```python
from build123d import *

# Parameters (mm, degrees)
F0_R      = 62.329716
F1_DEPTH  = 76.2
F2_R      = 33.756685
F3_DEPTH  = 50.8
F4_R      = 15.053655
F5_DEPTH  = 25.4
F6_R      = 16.209202
F7_DEPTH  = 25.4
F7_FACE_R = 16.209202
F8_DEPTH  = 254
F9_R      = 12.7
F10_SIZE  = 5.08


with BuildPart() as f1:
    # F0 (on Top) → F1 (new body)
    with BuildSketch(Plane.XY):
        with Locations((0, 5.263878)):
            Circle(F0_R)
    extrude(amount=F1_DEPTH)

    # F2 (on face) → F3 (join)
    with BuildSketch(Plane.XY.offset(76.2)):
        Circle(F2_R)
    extrude(amount=F3_DEPTH)

    # F4 (on face) → F5 (cut)
    with BuildSketch(Plane.XY.offset(127)):
        Circle(F4_R)
    extrude(amount=-F5_DEPTH, mode=Mode.SUBTRACT)

    # F6 (on face) → F7 (cut)
    with BuildSketch(Plane(origin=(0, 0, 0), x_dir=(1, 0, 0), z_dir=(0, 0, -1))):
        with Locations((0, -2.447213)):
            Circle(F6_R)
    extrude(amount=-F7_DEPTH, mode=Mode.SUBTRACT)

    # F7_face (on face) → F8 (cut)
    with BuildSketch(Plane(origin=(0, 2.447213, 25.4), x_dir=(1, 0, 0), z_dir=(0, 0, -1))):
        Circle(F7_FACE_R)
    extrude(amount=-F8_DEPTH, mode=Mode.SUBTRACT)

    # F9
    f9_edges = [f1.edges().sort_by_distance(p)[0] for p in [
        (-33.756685, 0, 127),
    ]]
    fillet(f9_edges, radius=F9_R)

    # F10
    f10_edges = [f1.edges().sort_by_distance(p)[0] for p in [
        (-62.329716, 5.263878, 76.2),
    ]]
    chamfer(f10_edges, length=F10_SIZE)


solid = f1.part
```
Read the model definition and answer for the solid it produces. Units are mm, in the model's axes. A direction names the side the tool comes from. Coordinates: 2 decimals unless noted, no trailing zeros. Order: outer loops, then holes, each group sorted by start corner. A loop starts at its lowest first (then second) coordinate and runs counter-clockwise, first axis right, second up. Notation, with made-up numbers: (-4.5, 81.5) - (22.5, 81.5) arc R12 cw to (22.5, 91.5) - close; hole circle Ø2 at (13, 14). An arc over 180 degrees is marked (long way). Answer as a JSON object with one key per item and string values. Group by question number.
Item 1: Section B-B (z = 78.5) is taken. Give the vertices of the cut face in (x, y).
Item 2: Section C-C (z = 11) is taken. Give the vertices of the cut face in (x, y).
Item 3: The mould has two halves that part along X. Classify faces 1 (the face through (-57.512, 7.795, 75.882)), 2 (the face through (-3.51, 18.27, 62.61)), 3 (the face through (-0.24, -15.05, 114.48)), 4 (the face through (-14, 32, 76.2)): +X half, -X half, draft (parallel to the pull), parting line (faces both ways), or undercut.
Item 4: Flat-ended cylindrical pins translate along their axes: P1, Ø5, axis at x = 11, y = 54, coming from the -Z side; P2, Ø10, axis at x = 5, z = 58, coming from the +Y side; P3, Ø6, axis at x = 44, z = 50.5, coming from the +Y side; P4, Ø8, axis at y = -19.5, z = 38, coming from the -X side. Find the tip coordinate at first contact, or state that the pin passes through.
Item 5: A tool of negligible diameter and unlimited length cuts with its end or side. For faces 5 (the face through (-7.318, -32.954, 94.983)), 6 (the face through (57.577, -18.609, 35.062)), from which of +Z, -Z, +X, -X, +Y, -Y can it reach the whole face along a straight path? Write none if from no direction.
Item 6: Section A-A (x = 0) is taken. Give the vertices of the cut face in (y, z).
Item 7: Consider probe 1 along Y at (x, z) = (0, 63); probe 2 along Y at (x, z) = (0, 83); probe 3 along Z at (x, y) = (11.5, 41.5). Determine where each line is inside the solid, lowest interval first. Write a range as from..to.
Results are:
{
 "1": {"outline": "circle Ø67.51 at (0, 0); hole circle Ø32.42 at (0, 2.45)"},
 "2": {"outline": "circle Ø124.66 at (0, 5.26); hole circle Ø32.42 at (0, 2.45)"},
 "3": {"face 1": "parting line", "face 2": "undercut", "face 3": "undercut", "face 4": "draft"},
 "4": {"P1": "stops at z = 0", "P2": "stops at y = 67.59", "P3": "stops at y = 52.21", "P4": "stops at x = -58.77"},
 "5": {"face 5": "+Z", "face 6": "+Z, -Z"},
 "6": {"outline": "(-57.07, 0) - (-13.76, 0) - (-13.76, 101.6) - (-15.05, 101.6) - (-15.05, 127) - (-21.06, 127) arc R12.7 ccw to (-33.76, 114.3) - (-33.76, 76.2) - (-51.99, 76.2) - (-57.07, 71.12) - close; (18.66, 0) - (67.59, 0) - (67.59, 71.12) - (62.51, 76.2) - (33.76, 76.2) - (33.76, 114.3) arc R12.7 ccw to (21.06, 127) - (18.66, 127) - close"},
 "7": {"probe 1": "y = -57.07..-13.76, 18.66..67.59", "probe 2": "y = -33.76..-13.76, 18.66..33.76", "probe 3": "z = 0..76.2"}
}
